from build123d import *

# Parameters (mm, degrees)
SKETCH_1_R          = 27
EXTRUDE_1_DEPTH     = 20
EXTRUDE_2_DEPTH     = 4
SKETCH_2_R          = 25
CUT_EXTRUDE_1_DEPTH = 8
SKETCH_3_R          = 23
CUT_EXTRUDE_2_DEPTH = 8
CUT_EXTRUDE_5_REACH = 50.518
SKETCH_8_R          = 5.1
CUT_EXTRUDE_6_REACH = 50.518
SKETCH_11_R         = 1.5
FILLET_1_R          = 10
FILLET_2_R          = 5
SKETCH_12_W         = 10
SKETCH_12_H         = 5
EXTRUDE_3_DEPTH     = 15
SKETCH_13_W         = 22
SKETCH_13_H         = 10
EXTRUDE_4_DEPTH     = 17
FILLET_3_R          = 10
FILLET_START        = -21.532998323
FILLET_4_DEPTH      = 0.497094834
FILLET_START_2      = -21.035903489
FILLET_4_2_DEPTH    = 12.502905266
FILLET_START_3      = -37
FILLET_4_3_DEPTH    = 74
FILLET_START_4      = -5
FILLET_4_4_DEPTH    = 10
CUT_EXTRUDE_7_REACH = 84.121
SKETCH_14_R         = 3
FILLET_5_R          = 5


with BuildPart() as part:
    # 草图1 → 凸台-拉伸1 (new body)
    with BuildSketch(Plane(origin=(0, 0, 0), x_dir=(0, 0, -1), z_dir=(1, 0, 0))):
        Circle(SKETCH_1_R)
    extrude(amount=EXTRUDE_1_DEPTH)

    # 草图10 → 凸台-拉伸2 (add)
    with BuildSketch(Plane.ZY):
        Polygon((0, 5), (37, 5), (37, -5), (0, -5), (-37, -5), (-37, 5), align=None)
    extrude(amount=-EXTRUDE_2_DEPTH)

    # 草图2 → 切除-拉伸1 (cut)
    with BuildSketch(Plane(origin=(20, 0, 0), x_dir=(0, 0, -1), z_dir=(1, 0, 0))):
        Circle(SKETCH_2_R)
    extrude(amount=-CUT_EXTRUDE_1_DEPTH, mode=Mode.SUBTRACT)

    # 草图3 → 切除-拉伸2 (cut)
    with BuildSketch(Plane(origin=(12, 0, 0), x_dir=(0, 0, -1), z_dir=(1, 0, 0))):
        Circle(SKETCH_3_R)
    extrude(amount=-CUT_EXTRUDE_2_DEPTH, mode=Mode.SUBTRACT)

    # 草图8 → 切除-拉伸5 (cut, up to next)
    with BuildSketch(Plane(origin=(4, 0, 0), x_dir=(0, 0, -1), z_dir=(1, 0, 0)), mode=Mode.PRIVATE) as cut_extrude_5_sk1:
        Circle(SKETCH_8_R)
    cut_extrude_5_tool1 = extrude(cut_extrude_5_sk1.sketch, amount=-CUT_EXTRUDE_5_REACH, mode=Mode.PRIVATE) & part.part
    add(cut_extrude_5_tool1.solids().sort_by_distance((4, 0, 0))[0], mode=Mode.SUBTRACT)

    # 草图11 → 切除-拉伸6 (cut, up to next)
    with BuildSketch(Plane(origin=(4, 0, 0), x_dir=(0, 0, -1), z_dir=(1, 0, 0)), mode=Mode.PRIVATE) as cut_extrude_6_sk1:
        with Locations((-33, 0)):
            Circle(SKETCH_11_R)
    cut_extrude_6_tool1 = extrude(cut_extrude_6_sk1.sketch, amount=-CUT_EXTRUDE_6_REACH, mode=Mode.PRIVATE) & part.part
    # 草图11 → 切除-拉伸6 (cut, up to next)
    with BuildSketch(Plane(origin=(4, 0, 0), x_dir=(0, 0, -1), z_dir=(1, 0, 0)), mode=Mode.PRIVATE) as cut_extrude_6_sk2:
        with Locations((33, 0)):
            Circle(SKETCH_11_R)
    cut_extrude_6_tool2 = extrude(cut_extrude_6_sk2.sketch, amount=-CUT_EXTRUDE_6_REACH, mode=Mode.PRIVATE) & part.part
    add(cut_extrude_6_tool1.solids().sort_by_distance((4, 0, 33))[0], mode=Mode.SUBTRACT)
    add(cut_extrude_6_tool2.solids().sort_by_distance((4, 0, -33))[0], mode=Mode.SUBTRACT)

    # 圆角1
    fillet_1_edges = [part.edges().sort_by_distance(p)[0] for p in [
        (2, 5, -26.532998323),
        (2, 5, 26.532998323),
        (2, -5, 26.532998323),
        (2, -5, -26.532998323),
    ]]
    fillet(fillet_1_edges, radius=FILLET_1_R)

    # 圆角2
    fillet_2_edges = [part.edges().sort_by_distance(p)[0] for p in [
        (2, 5, 37),
        (2, -5, 37),
        (2, -5, -37),
        (2, 5, -37),
    ]]
    fillet(fillet_2_edges, radius=FILLET_2_R)

    # 草图12 → 凸台-拉伸3 (add)
    with BuildSketch(Plane.ZY):
        with Locations((0, -24.032998323)):
            Rectangle(SKETCH_12_W, SKETCH_12_H)
    extrude(amount=EXTRUDE_3_DEPTH)

    # 草图13 → 凸台-拉伸4 (add)
    with BuildSketch(Plane.XZ.offset(26.532998323)):
        with Locations((-4, 0)):
            Rectangle(SKETCH_13_W, SKETCH_13_H)
    extrude(amount=EXTRUDE_4_DEPTH)

    # 圆角3
    fillet_3_edges = [part.edges().sort_by_distance(p)[0] for p in [
        (0, -24.032998323, -5),
        (0, -24.032998323, 5),
        (3.5, -26.532998323, -5),
        (3.5, -26.532998323, 5),
    ]]
    fillet(fillet_3_edges, radius=FILLET_3_R)

    # 圆角4: read off the stored shape, not the designer's step
    # 圆角4 outline → 圆角4 (add)
    with BuildSketch(Plane(origin=(0, 0, 0), x_dir=(1, 0, 0), z_dir=(0, 1, 0)).offset(FILLET_START)):
        with BuildLine():
            Line((0, -15), (0, -5))
            Line((0, -5), (-10, -5))
            ThreePointArc((-10, -5), (-2.928932188, -7.928932188), (0, -15))
        make_face()
        with BuildLine():
            ThreePointArc((0, 15), (-2.928932188, 7.928932188), (-10, 5))
            Line((-10, 5), (0, 5))
            Line((0, 5), (0, 15))
        make_face()
    extrude(amount=FILLET_4_DEPTH)

    # Fillet 4 2 outline → Fillet 4 2 (add)
    with BuildSketch(Plane(origin=(0, 0, 0), x_dir=(1, 0, 0), z_dir=(0, 1, 0)).offset(FILLET_START_2)):
        with BuildLine():
            Line((0, -15), (0, -5))
            Line((0, -5), (-10, -5))
            ThreePointArc((-10, -5), (-2.928932188, -7.928932188), (0, -15))
        make_face()
        with BuildLine():
            ThreePointArc((0, 15), (-2.928932188, 7.928932188), (-10, 5))
            Line((-10, 5), (0, 5))
            Line((0, 5), (0, 15))
        make_face()
    extrude(amount=FILLET_4_2_DEPTH)

    # Fillet 4 3 outline → Fillet 4 3 (cut)
    with BuildSketch(Plane.XY.offset(FILLET_START_3)):
        with BuildLine():
            Line((-15, -21.532998323), (-13, -21.532998323))
            add(Edge.make_bspline(
                [(-13, -21.532998323), (0, -21.532998323), (0, -8.532998323)],
                knots=[0, 0, 0, 1, 1, 1], degree=2, weights=[1, 0.707106781, 1]))
            Line((0, -8.532998323), (0, -7))
            Line((0, -7), (-15, -7))
            Line((-15, -7), (-15, -21.532998323))
        make_face()
    extrude(amount=FILLET_4_3_DEPTH, mode=Mode.SUBTRACT)

    # Fillet 4 4 outline → Fillet 4 4 (add)
    with BuildSketch(Plane.XY.offset(FILLET_START_4)):
        with BuildLine():
            add(Edge.make_bspline(
                [(-13, -21.532998323), (0, -21.532998323), (0, -8.532998323)],
                knots=[0, 0, 0, 1, 1, 1], degree=2, weights=[1, 0.707106781, 1]))
            Line((-13, -21.532998323), (0, -21.532998323))
            Line((0, -21.532998323), (0, -8.532998323))
        make_face()
    extrude(amount=FILLET_4_4_DEPTH)

    # 草图14 → 切除-拉伸7 (cut, up to next)
    with BuildSketch(Plane(origin=(0, -43.532998323, 0), x_dir=(-1, 0, 0), z_dir=(0, -1, 0)), mode=Mode.PRIVATE) as cut_extrude_7_sk1:
        with Locations(Location((9, 0, 0), (0, 0, 90))):
            Circle(SKETCH_14_R)
    cut_extrude_7_tool1 = extrude(cut_extrude_7_sk1.sketch, amount=-CUT_EXTRUDE_7_REACH, mode=Mode.PRIVATE) & part.part
    add(cut_extrude_7_tool1.solids().sort_by_distance((-9, -43.532998, 0))[0], mode=Mode.SUBTRACT)

    # 圆角5
    # the kernel refuses this fillet: 5 mm, written as the material it takes off along each edge
    with BuildSketch(Plane(origin=(7, -33.823069051, -15), x_dir=(0, 0, 1), z_dir=(0, -1, 0))) as fillet_5_piece_1_section:
        with BuildLine():
            CenterArc((10 + FILLET_5_R, FILLET_5_R), FILLET_5_R, 180, 90)
            Line((10 + FILLET_5_R, 0), (10, 0))
            Line((10, 0), (10, FILLET_5_R))
        make_face()
    fillet_5_piece_1 = revolve(axis=Axis((7, -33.823069051, -15), (-1, 0, 0)), revolution_arc=137.718699106, mode=Mode.PRIVATE)
    fillet_5_piece_1 = fillet_5_piece_1 - Plane(origin=(7, 0, 0), x_dir=(0, 0, -1), z_dir=(-1, 0, 0)) * Cylinder(27, 60, mode=Mode.PRIVATE)
    add(fillet_5_piece_1, mode=Mode.SUBTRACT)
    with BuildSketch(Plane(origin=(7, -33.823069051, 15), x_dir=(0, 0, -1), z_dir=(0, -1, 0))) as fillet_5_piece_2_section:
        with BuildLine():
            CenterArc((10 + FILLET_5_R, -FILLET_5_R), FILLET_5_R, 90, 90)
            Line((10 + FILLET_5_R, 0), (10, 0))
            Line((10, 0), (10, -FILLET_5_R))
        make_face()
    fillet_5_piece_2 = revolve(axis=Axis((7, -33.823069051, 15), (1, 0, 0)), revolution_arc=137.718699106, mode=Mode.PRIVATE)
    fillet_5_piece_2 = fillet_5_piece_2 - Plane(origin=(7, 0, 0), x_dir=(0, 0, -1), z_dir=(-1, 0, 0)) * Cylinder(27, 60, mode=Mode.PRIVATE)
    add(fillet_5_piece_2, mode=Mode.SUBTRACT)
    with BuildSketch(Plane(origin=(7, -33.823069051, -5), x_dir=(-1, 0, 0), z_dir=(0, -1, 0))) as fillet_5_piece_3:
        with BuildLine():
            CenterArc((FILLET_5_R, -FILLET_5_R), FILLET_5_R, 90, 90)
            Line((0, -FILLET_5_R), (0, 0))
            Line((0, 0), (FILLET_5_R, 0))
        make_face()
    extrude(amount=22.209929272, mode=Mode.SUBTRACT)
    with BuildSketch(Plane(origin=(7, -33.823069051, 5), x_dir=(-1, 0, 0), z_dir=(0, -1, 0))) as fillet_5_piece_4:
        with BuildLine():
            CenterArc((FILLET_5_R, FILLET_5_R), FILLET_5_R, 180, 90)
            Line((0, FILLET_5_R), (0, 0))
            Line((0, 0), (FILLET_5_R, 0))
        make_face()
    extrude(amount=22.209929272, mode=Mode.SUBTRACT)
    with BuildSketch(Plane(origin=(-15, -9.032998323, 5), x_dir=(1, 0, 0), z_dir=(0, -1, 0)), Plane(origin=(-15, -56.032998323, -5), x_dir=(1, 0, 0), z_dir=(0, 1, 0))) as fillet_5_piece_5:
        with BuildLine():
            CenterArc((FILLET_5_R, -FILLET_5_R), FILLET_5_R, 90, 90)
            Line((0, -FILLET_5_R), (0, 0))
            Line((0, 0), (FILLET_5_R, 0))
        make_face()
    extrude(amount=47, mode=Mode.SUBTRACT)


solid = part.part
Source: CAD feature listing. Evaluate the final solid. Frame: model axes, mm. A direction names the side the tool comes from. Give positions to 0.01 mm unless a question says otherwise; leave off trailing zeros. Order: outer loops, then holes, each group sorted by start corner. A loop starts at its lowest first (then second) coordinate and runs counter-clockwise, first axis right, second up. Notation, with made-up numbers: (83, 77.5) -> (136, 77.5) arc R13 cw to (136, 90.5) -> close; hole circle Ø9 at (47, 2.5). An arc over 180 degrees is marked (long way). Write item = value, one per line.
Item 1: Set-up query: faces 1 (the face through (-4, -39, 5)), 2 (the face through (-4, -39, -5)), 3 (the face through (12, -7.3, -22.1)), 4 (the face through (-14, -21.533, 0)), 5 (the face through (7, -39, 0)). Return all of +Z, -Z, +X, -X, +Y, -Y with unobstructed straight access to the full face (end or side cutting, diameter ignored); none if empty.
Check result:
face_1 = +Z, +X, -X, -Y
face_2 = -Z, +X, -X, -Y
face_3 = +X
face_4 = +Z, -Z, -X, +Y
face_5 = +X, -Y
Item 2: Section query A-A (x = 5.5). Output: boundary loops of the cut face in (y, z).
Check result:
outline = (-43.53, -3.57) -> (-33.82, -3.57) arc R11.43 cw to (-26.21, -6.47) arc R27 ccw (long way) to (-26.21, 6.47) arc R11.43 cw to (-33.82, 3.57) -> (-43.53, 3.57) -> close; hole circle Ø46 at (0, 0)
Item 3: Contact query for flat-ended pins moving along their axis: pin 1 (8 mm diameter, centred on x = 12, y = -20, fed in from -Z); pin 2 (4 mm diameter, centred on x = 8.5, y = 16.5, fed in from -Z); pin 3 (0.6 mm diameter, centred on x = -14.5, z = 1, fed in from +Y). Output: stop coordinate, or through.
Check result:
pin_1 = -21.75
pin_2 = -22.78
pin_3 = -21.53
Item 4: Mould query, pull axis Y, two halves, no side actions, for faces 6 (the face through (4, 0, -31)), 7 (the face through (1.97, 6.92, 27.93)), 8 (the face through (4, 5.4, 0.3)). Classes: +Y half, -Y half, draft (parallel to the pull), parting line (faces both ways), or undercut.
Check result:
face_6 = draft
face_7 = +Y half
face_8 = undercut
Item 5: Ray query, probe 1 along Y at (x, z) = (2, 0); probe 2 along Y at (x, z) = (2.05, 33); probe 3 along Z at (x, y) = (-9, -38.25). Return the intervals inside material, ascending.
Check result:
probe_1 = -43.53 to -5.1, 5.1 to 27
probe_2 = -5.01 to -1.5, 1.5 to 5.01
probe_3 = -5 to -3, 3 to 5
